The model under review builds one solid part; all positions refer to its coordinate system, in mm. Face numbers are marked on the shaded views. A direction names the side the tool comes from. Coordinates: 2 decimals unless noted, no trailing zeros. Loops run counter-clockwise (first coordinate to the right, second up) from the corner with the lowest first, then second, coordinate; pieces in that order, holes last. Notation, with made-up numbers: (58, -16.5) - (116, -16.5) arc R23 ccw to (116, 15.5) - close; hole circle Ø8 at (48.25, -39.5). An arc over 180 degrees is marked (long way). Answer in a Markdown table with one row per item. Add a question column.
(1) Machinability: for the marked faces 1, 2 and 3, which of the approach directions +Z, -Z, +X, -X, +Y, -Y give a long, thin tool a straight path to every point of the face, cutting with its end or side? Answer none if there is none.
(2) We need section D-D on x = 11. Write out the cut boundary in (y, z).
(3) We need section C-C on y = -5.35. Write out the cut boundary in (x, z).
(4) We need section A-A on y = -7.25. Write out the cut boundary in (x, z), plus the area to 3 significant figures.
(5) For line 1 along Y through (x, z) = (12.75, 6.95); line 2 along Z through (x, y) = (14.25, -5.1); line 3 along X through (y, z) = (-6.95, 6.05), list the stretches that pass through material, from the lowest coordinate up.
(6) For P1, Ø2.5, axis at x = 9.12, y = -4.91, coming from the -Z side; P2, Ø2, axis at x = 8.5, y = -4.5, coming from the +Z side; P3, Ø1.1, axis at y = -7.5, z = 5.5, coming from the -X side; P4, Ø2.5, axis at x = 11.12, z = 7.44, coming from the +Y side, all flat-tipped, find the tip position at first contact; note any pin that passes through.
(7) We need section B-B on z = 7.7. Write out the cut boundary in (x, y).
(8) Mouldability with a two-part tool opening along Y and no side actions: class the marked faces 4, 5 and 6 as +Y half, -Y half, draft (parallel to the pull), parting line (faces both ways), or undercut.
from build123d import *

# Parameters (mm, degrees)
SKETCH_1_R      = 5
EXTRUDE_1_DEPTH = 5
EXTRUDE_START   = -15
SKETCH_2_R      = 5
EXTRUDE_2_DEPTH = 5
SCALE_1_SCALE   = 0.2


with BuildPart() as part:
    # 草圖1 → 填料-伸長1 (new body)
    with BuildSketch(Plane.XY):
        with BuildLine():
            Line((0, 10), (15, 10))
            Line((15, 10), (35, -10))
            Line((35, -10), (35, -15))
            Line((35, -15), (0, -15))
            Line((0, -15), (0, -10))
            ThreePointArc((0, -10), (-10, 0), (0, 10))
        make_face()
        Circle(SKETCH_1_R, mode=Mode.SUBTRACT)
    extrude(amount=EXTRUDE_1_DEPTH)

    # 草圖2 → 填料-伸長2 (add)
    with BuildSketch(Plane(origin=(0, 0, 0), x_dir=(1, 0, 0), z_dir=(0, 1, 0)).offset(EXTRUDE_START)):
        with BuildLine():
            Line((0, -15), (0, -5))
            Line((0, -5), (20, -5))
            Line((20, -5), (20, -15))
            ThreePointArc((20, -15), (10, -25), (0, -15))
        make_face()
        with Locations((10, -15)):
            Circle(SKETCH_2_R, mode=Mode.SUBTRACT)
    extrude(amount=EXTRUDE_2_DEPTH)


with BuildPart() as part_1:
    # 縮放比例1: scaled about (11.398892544, -6.138978205, 5.550553728)
    add(part.part.scale(SCALE_1_SCALE).moved(Location((9.119114035, -4.911182564, 4.440442982))))


solid = part_1.part
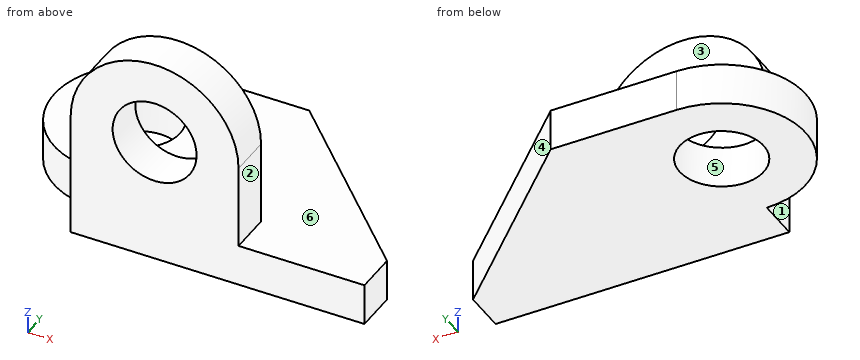
Outcome:
| question | item | result |
|---|---|---|
| 1 | face 1 | +Z, -Z, -X, -Y |
| 1 | face 2 | +Z, +X, +Y, -Y |
| 1 | face 3 | +Z, +X, -X, +Y |
| 2 | outline | (-7.91, 4.44) - (-2.91, 4.44) - (-2.91, 5.44) - (-6.91, 5.44) - (-6.91, 6.45) - (-7.91, 6.45) - close; (-7.91, 8.43) - (-6.91, 8.43) - (-6.91, 9.44) - (-7.91, 9.44) - close |
| 3 | outline | (7.17, 4.44) - (8.22, 4.44) - (8.22, 5.44) - (7.17, 5.44) - close; (10.02, 4.44) - (14.56, 4.44) - (14.56, 5.44) - (10.02, 5.44) - close |
| 4 | outline | (9.12, 4.44) - (16.12, 4.44) - (16.12, 5.44) - (13.12, 5.44) - (13.12, 7.44) arc R2 ccw to (9.12, 7.44) - close; hole circle Ø2 at (11.12, 7.44) |
| 4 | area | 18.1 mm² |
| 5 | line 1 | -7.91 to -6.91 |
| 5 | line 2 | 4.44 to 5.44 |
| 5 | line 3 | 9.12 to 13.12 |
| 6 | P1 | z = 4.44 |
| 6 | P2 | z = 5.44 |
| 6 | P3 | x = 9.12 |
| 6 | P4 | y = -6.91 |
| 7 | outline | (9.14, -7.91) - (10.15, -7.91) - (10.15, -6.91) - (9.14, -6.91) - close; (12.08, -7.91) - (13.1, -7.91) - (13.1, -6.91) - (12.08, -6.91) - close |
| 8 | face 4 | +Y half |
| 8 | face 5 | undercut |
| 8 | face 6 | draft |
